```python
from build123d import *

# Parameters (mm, degrees)
F1_DEPTH = 40
F2_W     = 6.804615
F2_H     = 50.8
F3_DEPTH = 39.5


with BuildPart() as f1:
    # F0 (on Right) → F1 (new body)
    with BuildSketch(Plane.YZ):
        with BuildLine():
            Line((-38.531435, 21.988993), (-38.531435, -18.011007))
            ThreePointArc((-38.531435, -18.011007), (-37.781435, -18.761007), (-37.031435, -18.011007))
            Line((-37.031435, -18.011007), (-37.031435, 21.988993))
            ThreePointArc((-37.031435, 21.988993), (-40.567433, 25.488808), (-44.030694, 21.917))
            Line((-44.030694, 21.917), (-41.336774, -9.982696))
            Line((-41.336774, -9.982696), (-41.336774, -18.011007))
            ThreePointArc((-41.336774, -18.011007), (-40.584104, -18.763676), (-39.831435, -18.011007))
            Line((-39.831435, -18.011007), (-39.831435, -9.982696))
            Line((-39.831435, -9.982696), (-42.531435, 21.988993))
            ThreePointArc((-42.531435, 21.988993), (-40.531435, 23.988993), (-38.531435, 21.988993))
        make_face()
    extrude(amount=F1_DEPTH)

    # F2 (on Front) → F3 (cut)
    with BuildSketch(Plane.XZ):
        with Locations((20.661171, -3.411007)):
            Rectangle(F2_W, F2_H)
    extrude(amount=F3_DEPTH, mode=Mode.SUBTRACT)


solid = f1.part
```
Check sheet for the modelled part. Datum: model origin and axes. Units: mm. A direction names the side the tool comes from. Coordinates: 2 decimals unless noted, no trailing zeros. Order: outer loops, then holes, each group sorted by start corner. A loop starts at its lowest first (then second) coordinate and runs counter-clockwise, first axis right, second up. Notation, with made-up numbers: M 10,-23.5 L 63,-23.5 A33 ccw 63,8.5 Z; hole C 34.5,71 d5. An arc over 180 degrees is marked long. One line per question, with ' | ' between items. Start each with the question number.
Item 1: Sectioned sample at D-D on z = -8.5. Record the cut outline in (x, y), and give its area (3 significant figures).
Item 2: Sectioned sample at A-A on y = -40.75. Record the cut outline in (x, z).
Item 3: Sectioned sample at C-C on z = 22.5. Record the cut outline in (x, y).
Item 4: Sectioned sample at B-B on x = 15. Record the cut outline in (y, z).
Item 5: Gauge pin test, flat ends, axial feed: P1, Ø14, axis at x = 4.5, z = 1, coming from the -Y side; P2, Ø2, axis at x = 11.5, y = -41, coming from the +Z side; P3, Ø3, axis at x = 6, y = -38, coming from the +Z side; P4, Ø9, axis at x = 15, z = -14.5, coming from the -Y side. Record the tip position at first contact, or that the pin passes through.
Item 6: Material ranges on line 1 (Y direction, x = 35.5, z = -10); line 2 (X direction, y = -37.25, z = -15); line 3 (Y direction, x = 5, z = 2), recorded low to high.
Item 7: Mould release check, pull along Z, two halves, no side actions. Record for faces 6 (the flat face through (19.72, -41.163, 5.779)), 7 (the flat face through (0, -38, 4)), 8 (the cylindrical face through (8.51, -37.8, -18.76)): pulls with the +Z half, pulls with the -Z half, needs draft (parallel to the pull), parting line crosses it, or undercut.
Item 8: Access from +Z, -Z, +X, -X, +Y, -Y to the whole of each face (thin tool, end or side, straight path). Record for faces 1 (the flat face through (17.259, -38, 1)), 2 (the flat face through (9, -38.531, 2)), 3 (the flat face through (20, -41.337, -14)), 4 (the cylindrical face through (19.72, -40.58, 23.99)), 5 (the flat face through (9, -37.031, 2)).
Answer below:
1) outline: M 0,-41.46 L 40,-41.46 L 40,-39.96 L 0,-39.96 Z; M 0,-38.53 L 17.26,-38.53 L 17.26,-37.03 L 0,-37.03 Z; M 24.06,-38.53 L 40,-38.53 L 40,-37.03 L 24.06,-37.03 Z | area: 110 mm^2
2) outline: M 0,-18.75 L 40,-18.75 L 40,0.89 L 0,0.89 Z; M 0,23.98 L 40,23.98 L 40,25.48 L 0,25.48 Z
3) outline: M 0,-43.99 L 40,-43.99 L 40,-42.47 L 0,-42.47 Z; M 0,-38.6 L 40,-38.6 L 40,-37.07 L 0,-37.07 Z
4) outline: M -44.03,21.92 L -41.34,-9.98 L -41.34,-18.01 A0.75 ccw -39.83,-18.01 L -39.83,-9.98 L -42.53,21.99 A2 cw -38.53,21.99 L -38.53,-18.01 A0.75 ccw -37.03,-18.01 L -37.03,21.99 A3.5 ccw long Z
5) P1: stops at y = -42.86 | P2: stops at z = 25.49 | P3: stops at z = 25.33 | P4: stops at y = -41.34
6) line 1: y = -41.34 to -39.83, -38.53 to -37.03 | line 2: x = 0 to 17.26, 24.06 to 40 | line 3: y = -42.35 to -40.84, -38.53 to -37.03
7) face 6: undercut | face 7: needs draft | face 8: pulls with the -Z half
8) face 1: -Z, +Y | face 2: -Z, +X, -X | face 3: -Z, +X, -X, -Y | face 4: +X, -X | face 5: +Z, -Z, +X, -X, +Y
